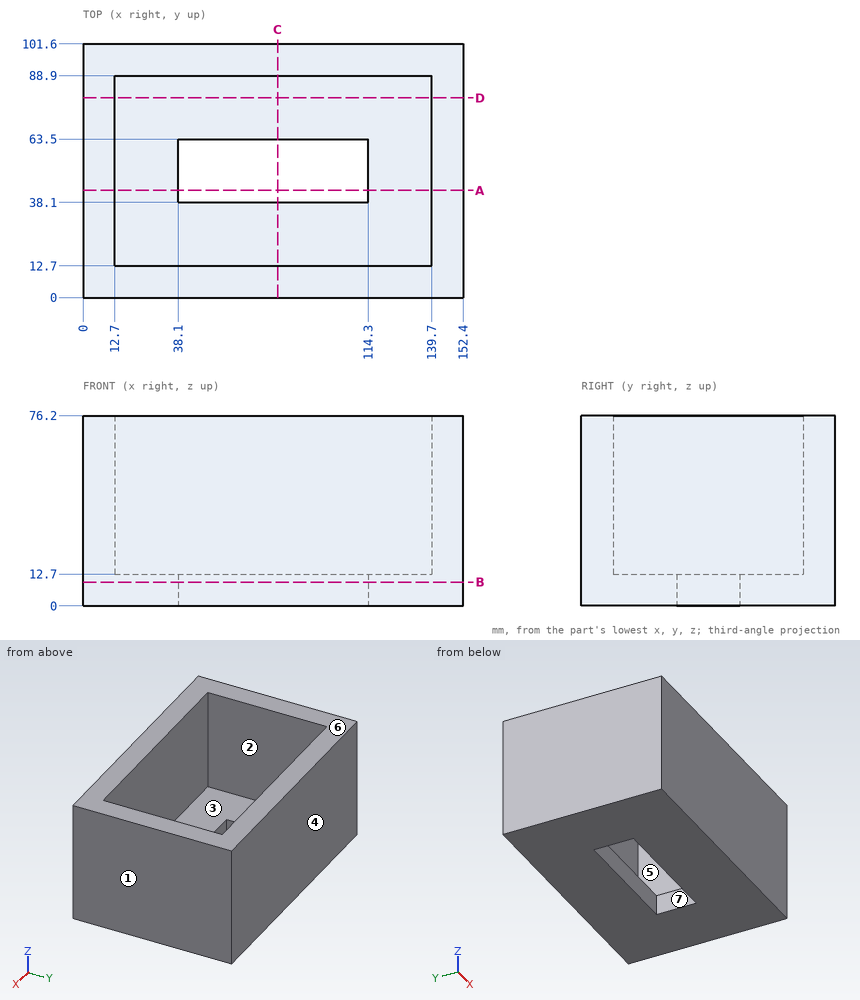
For this review, use the dimensioned drawing (mm, ordinates from the lowest corner) and the shaded views. A direction names the side the tool comes from. Give positions to 0.01 mm unless a question says otherwise; leave off trailing zeros. Write each loop counter-clockwise with the first axis right and the second up, starting at its lowest first coordinate (ties: lowest second). Pieces come first, ordered by that corner, then holes. Notation, with made-up numbers: M 7,18.25 L 57,18.25 A29 ccw 57,43.25 Z; hole C 26.5,-27 d1. An arc over 180 degrees is marked long. Answer as a JSON object with one key per item and string values. Group by question number.
Item 1: Consider section C-C on x = 78. Write out the cut boundary in (y, z).
Item 2: Consider section A-A on y = 43. Write out the cut boundary in (x, z).
Item 3: Draft analysis for pull direction X (two halves, no side actions). For the marked faces 1, 2, 3 and 4, state which applies: +X half, -X half, draft (parallel to the pull), parting line (faces both ways), or undercut.
Item 4: Consider section D-D on y = 80. Write out the cut boundary in (x, z).
Item 5: Tool access review of the marked faces 5, 6 and 7: name each direction out of +Z, -Z, +X, -X, +Y, -Y from which nothing blocks a thin tool from reaching the whole face with its end or side.
Item 6: For pin 1 Ø4 at (x, y) = (59, 13) entering from +Z; pin 2 Ø3 at (x, y) = (21.5, 80.5) entering from +Z, all flat-tipped, find the tip position at first contact; note any pin that passes through.
Item 7: For probe 1 along Y at (x, z) = (87.5, 73); probe 2 along X at (y, z) = (88, 58); probe 3 along Z at (x, y) = (16, 25), list the stretches that pass through material, from the lowest coordinate up. Write a range as [from, to].
Item 8: Consider section B-B on z = 9.5. Write out the cut boundary in (x, y), plus the area to 3 significant figures.
Check result:
{
 "1": {"outline": "M 0,0 L 38.1,0 L 38.1,12.7 L 12.7,12.7 L 12.7,76.2 L 0,76.2 Z; M 63.5,0 L 101.6,0 L 101.6,76.2 L 88.9,76.2 L 88.9,12.7 L 63.5,12.7 Z"},
 "2": {"outline": "M 0,0 L 38.1,0 L 38.1,12.7 L 12.7,12.7 L 12.7,76.2 L 0,76.2 Z; M 114.3,0 L 152.4,0 L 152.4,76.2 L 139.7,76.2 L 139.7,12.7 L 114.3,12.7 Z"},
 "3": {"face 1": "+X half", "face 2": "undercut", "face 3": "undercut", "face 4": "draft"},
 "4": {"outline": "M 0,0 L 152.4,0 L 152.4,76.2 L 139.7,76.2 L 139.7,12.7 L 12.7,12.7 L 12.7,76.2 L 0,76.2 Z"},
 "5": {"face 5": "+Z", "face 6": "+Z, +X, -X, +Y, -Y", "face 7": "+Z, -Z"},
 "6": {"pin 1": "stops at z = 76.2", "pin 2": "stops at z = 12.7"},
 "7": {"probe 1": "y = [0, 12.7], [88.9, 101.6]", "probe 2": "x = [0, 12.7], [139.7, 152.4]", "probe 3": "z = [0, 12.7]"},
 "8": {"outline": "M 0,0 L 152.4,0 L 152.4,101.6 L 0,101.6 Z; hole M 38.1,38.1 L 114.3,38.1 L 114.3,63.5 L 38.1,63.5 Z", "area": "13,500 mm^2"}
}
